```python
from build123d import *

# Parameters (mm, degrees)
BASE_FLANGE1_DEPTH         = 65
F_6_6_6_6_DIAMETER_HOLE1_D = 6.6
BREAK_CORNER1_DEPTH        = 3.175


# Read off the part's stored shape, not the designer's step: Break-Corner1
# Sheet-metal steps are written as plain solids
with BuildPart() as part:
    # Sketch1 → Base-Flange1 (new, symmetric)
    with BuildSketch(Plane.XY):
        with BuildLine():
            Line((-100, 0), (-56.35, 0))
            ThreePointArc((-56.35, 0), (-51.859871939, 1.859871939), (-50, 6.35))
            Line((-50, 6.35), (-50, 160))
            ThreePointArc((-50, 160), (0, 210), (50, 160))
            Line((50, 160), (50, 6.35))
            ThreePointArc((50, 6.35), (51.859871939, 1.859871939), (56.35, 0))
            Line((56.35, 0), (100, 0))
            Line((100, 0), (100, 3.175))
            Line((100, 3.175), (56.35, 3.175))
            ThreePointArc((56.35, 3.175), (54.10493597, 4.10493597), (53.175, 6.35))
            Line((53.175, 6.35), (53.175, 160))
            ThreePointArc((53.175, 160), (0, 213.175), (-53.175, 160))
            Line((-53.175, 160), (-53.175, 6.35))
            ThreePointArc((-53.175, 6.35), (-54.10493597, 4.10493597), (-56.35, 3.175))
            Line((-56.35, 3.175), (-100, 3.175))
            Line((-100, 3.175), (-100, 0))
        make_face()
    extrude(amount=BASE_FLANGE1_DEPTH, both=True)

    # Ø6.6 (6.6) Diameter Hole1 (through all)
    with Locations(Plane(origin=(0, 3.175, 0), x_dir=(1, 0, 0), z_dir=(0, 1, 0))):
        with Locations((-80, 0), (80, 0)):
            Hole(F_6_6_6_6_DIAMETER_HOLE1_D / 2)

    # Break-Corner1 outline → Break-Corner1 (cut)
    with BuildSketch(Plane(origin=(0, 0, 0), x_dir=(1, 0, 0), z_dir=(0, 1, 0))):
        Polygon((-100, -65), (-95, -65), (-100, -60), align=None)
        Polygon((-100, 65), (-100, 60), (-95, 65), align=None)
        Polygon((100, -65), (100, -60), (95, -65), align=None)
        Polygon((95, 65), (100, 60), (100, 65), align=None)
    extrude(amount=BREAK_CORNER1_DEPTH, mode=Mode.SUBTRACT)


solid = part.part
```
Source: CAD feature listing. Evaluate the final solid. Frame: model axes, mm. A direction names the side the tool comes from. Give positions to 0.01 mm unless a question says otherwise; leave off trailing zeros. Write each loop counter-clockwise with the first axis right and the second up, starting at its lowest first coordinate (ties: lowest second). Pieces come first, ordered by that corner, then holes. Notation, with made-up numbers: (12, 85.25) - (36, 85.25) arc R24 cw to (36, 118.25) - close; hole circle Ø5 at (40, 69). An arc over 180 degrees is marked (long way). One line per item, written item: value. Start each with the question number.
Q1. First-contact query: pin 1 Ø12 at (x, z) = (40, -20.5) entering from -Y; pin 2 Ø3 at (x, z) = (76.5, 32) entering from +Y (3 decimals); pin 3 Ø4 at (y, z) = (59, -14) entering from +X (3 decimals). Flat tips, straight axial feed; report the tip coordinate or a pass-through.
Q2. Draft query along X for faces 1 (the face through (-50, 82, 1)), 2 (the face through (1.169, 213.162, 0.91)), 3 (the face through (73, 0, 1)). Return one class per face: +X half, -X half, draft (parallel to the pull), parting line (faces both ways), or undercut.
Q3. Section query C-C, the plane y = 78. Return the cut outline in (x, z) (3 decimals).
Q4. Section query D-D, the plane z = -42.5. Return the cut outline in (x, y) (3 decimals).
Q5. Material intervals for probe 1 along X at (y, z) = (84.5, 5) (3 decimals); probe 2 along Z at (x, y) = (80, 1.05); probe 3 along Y at (x, z) = (67.5, 59.5) (3 decimals), sorted ascending. Write a range as from..to.
Q6. Set-up query: faces 4 (the face through (53.175, 82, 1)), 5 (the face through (51.81, 1.91, 0.91)), 6 (the face through (-53.175, 84, 1)), 7 (the face through (-83.33, 0, 0.91)). Return all of +Z, -Z, +X, -X, +Y, -Y with unobstructed straight access to the full face (end or side cutting, diameter ignored); none if empty.
Q7. Section query B-B, the plane z = 0. Return the cut outline in (x, y) (3 decimals), then the cut area to 3 significant figures.
Q8. Section query A-A, the plane x = -80. Return the cut outline in (y, z) (3 decimals).
Answer:
1. pin 1: stops at y = 179.6
1. pin 2: stops at y = 3.175
1. pin 3: stops at x = 53.175
2. face 1: undercut
2. face 2: parting line
2. face 3: draft
3. outline: (-53.175, -65) - (-50, -65) - (-50, 65) - (-53.175, 65) - close; (50, -65) - (53.175, -65) - (53.175, 65) - (50, 65) - close
4. outline: (-100, 0) - (-56.35, 0) arc R6.35 ccw to (-50, 6.35) - (-50, 160) arc R50 cw to (50, 160) - (50, 6.35) arc R6.35 ccw to (56.35, 0) - (100, 0) - (100, 3.175) - (56.35, 3.175) arc R3.175 cw to (53.175, 6.35) - (53.175, 160) arc R53.175 ccw to (-53.175, 160) - (-53.175, 6.35) arc R3.175 cw to (-56.35, 3.175) - (-100, 3.175) - close
5. probe 1: x = -53.175..-50, 50..53.175
5. probe 2: z = -65..-3.3, 3.3..65
5. probe 3: y = 0..3.175
6. face 4: +Z, -Z, +X, +Y
6. face 5: +Z, -Z, -Y
6. face 6: +Z, -Z, -X, +Y
6. face 7: +Z, -Z, +X, -X, -Y
7. outline: (-100, 0) - (-83.3, 0) - (-83.3, 3.175) - (-100, 3.175) - close; (-76.7, 0) - (-56.35, 0) arc R6.35 ccw to (-50, 6.35) - (-50, 160) arc R50 cw to (50, 160) - (50, 6.35) arc R6.35 ccw to (56.35, 0) - (76.7, 0) - (76.7, 3.175) - (56.35, 3.175) arc R3.175 cw to (53.175, 6.35) - (53.175, 160) arc R53.175 ccw to (-53.175, 160) - (-53.175, 6.35) arc R3.175 cw to (-56.35, 3.175) - (-76.7, 3.175) - close; (83.3, 0) - (100, 0) - (100, 3.175) - (83.3, 3.175) - close
7. area: 1,770 mm2
8. outline: (0, -65) - (3.175, -65) - (3.175, -3.3) - (0, -3.3) - close; (0, 3.3) - (3.175, 3.3) - (3.175, 65) - (0, 65) - close
